Source: CAD feature listing. Evaluate the final solid. Frame: model axes, mm. A direction names the side the tool comes from. Give positions to 0.01 mm unless a question says otherwise; leave off trailing zeros. Loops run counter-clockwise (first coordinate to the right, second up) from the corner with the lowest first, then second, coordinate; pieces in that order, holes last. Notation, with made-up numbers: M 48,-15.75 L 104,-15.75 A17 cw 104,15.25 Z; hole C 47.25,44 d9. An arc over 180 degrees is marked long. Answer in a Markdown table with one row per item.
```python
from build123d import *

# Parameters (mm, degrees)
F1_DEPTH = 600


with BuildPart() as f1:
    # F0 (on Top) → F1 (new body)
    with BuildSketch(Plane.XY):
        Polygon((0, 70), (0, 0), (70, 0), (70, 50), (100, 50), (100, 100), (50, 100), (50, 70), align=None)
    extrude(amount=F1_DEPTH)


with BuildPart() as f2_1:
    # F2: copy of F1
    add(f1.part)


solid = f1.part
```
1) Section A-A, the plane z = 532. Return loops of the section in (x, y).
Reply:
| item | result |
|---|---|
| outline | M 0,0 L 70,0 L 70,50 L 100,50 L 100,100 L 50,100 L 50,70 L 0,70 Z |
2) Pull-direction query (Z, two-part tool) for faces 4 (the flat face through (49, 51, 0)), 5 (the flat face through (0, 35, 296)), 6 (the flat face through (49, 51, 600)); classes: released by +Z, released by -Z, zero draft, split by the parting line, or undercut.
Reply:
| item | result |
|---|---|
| face 4 | released by -Z |
| face 5 | zero draft |
| face 6 | released by +Z |
3) Set-up query: faces 1 (the flat face through (85, 50, 296)), 2 (the flat face through (25, 70, 296)), 3 (the flat face through (35, 0, 296)). Return all of +Z, -Z, +X, -X, +Y, -Y with unobstructed straight access to the full face (end or side cutting, diameter ignored); none if empty.
Reply:
| item | result |
|---|---|
| face 1 | +Z, -Z, +X, -Y |
| face 2 | +Z, -Z, -X, +Y |
| face 3 | +Z, -Z, +X, -X, -Y |
4) Pin query (flat end, axial travel): pin 1 Ø15 at (y, z) = (91.5, 362.5) entering from -X; pin 2 Ø6 at (y, z) = (16.5, 474.5) entering from +X; pin 3 Ø25 at (x, z) = (30, 360.5) entering from +Y. Return the tip coordinate at first contact, or that it passes through.
Reply:
| item | result |
|---|---|
| pin 1 | stops at x = 50 |
| pin 2 | stops at x = 70 |
| pin 3 | stops at y = 70 |
5) Section B-B, the plane y = 25.5. Return loops of the section in (x, z), then the cut area to 3 significant figures.
Reply:
| item | result |
|---|---|
| outline | M 0,0 L 70,0 L 70,600 L 0,600 Z |
| area | 42,000 mm² |
6) Material intervals for L1, parallel to X at y = 17.5, z = 328; L2, parallel to X at y = 82.5, z = 386, sorted ascending.
Reply:
| item | result |
|---|---|
| L1 | x = 0 to 70 |
| L2 | x = 50 to 100 |
